Can you work these out from the model? Positions are in its coordinate system, mm. Coordinates: 2 decimals unless noted, no trailing zeros. Write each loop counter-clockwise with the first axis right and the second up, starting at its lowest first coordinate (ties: lowest second). Pieces come first, ordered by that corner, then holes. Notation, with made-up numbers: M 17.25,77.25 L 75.25,77.25 A20 cw 75.25,88.25 Z; hole C 89.25,12.5 d4. An arc over 180 degrees is marked long. Answer as a JSON object with one key per item and string values. Group by question number.
from build123d import *

# Parameters (mm, degrees)
F0_W     = 114.3
F0_H     = 844.55
F0_H_2   = 1968.5
F0_W_2   = 571.5
F0_H_3   = 25.4
F1_DEPTH = 3.175


with BuildPart() as f1:
    # F0 (on Front) → F1 (new body)
    with BuildSketch(Plane.XZ):
        Polygon((-901.7, 0), (0, 0), (0, 2019.3), (-901.7, 2019.3), (-901.7, 1136.65), (-749.3, 1136.65), (-749.3, 882.65), (-901.7, 882.65), align=None)
        with Locations((-819.15, 447.675)):
            Rectangle(F0_W, F0_H, mode=Mode.SUBTRACT)
        Polygon((-736.6, 1354.93125), (-736.6, 1993.9), (-165.1, 1993.9), (-165.1, 1354.93125), (-165.1, 1329.53125), (-165.1, 689.76875), (-165.1, 664.36875), (-165.1, 25.4), (-736.6, 25.4), (-736.6, 664.36875), (-736.6, 689.76875), (-736.6, 1329.53125), align=None, mode=Mode.SUBTRACT)
        with Locations((-819.15, 1571.625)):
            Rectangle(F0_W, F0_H, mode=Mode.SUBTRACT)
        with Locations((-82.55, 1009.65)):
            Rectangle(F0_W, F0_H_2, mode=Mode.SUBTRACT)
        with Locations((-450.85, 1342.23125)):
            Rectangle(F0_W_2, F0_H_3)
        with Locations((-450.85, 677.06875)):
            Rectangle(F0_W_2, F0_H_3)
    extrude(amount=F1_DEPTH)


solid = f1.part
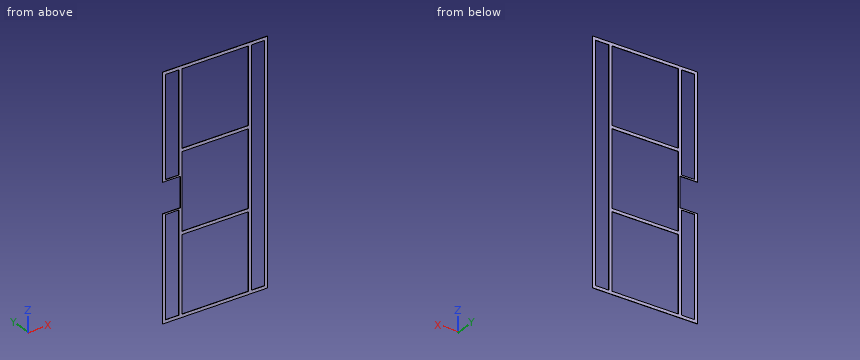
Q1. Please list where these lines run through material, in increasing order: L1, parallel to X at y = -1.6, z = 143; L2, parallel to X at y = -1.1, z = 893; L3, parallel to X at y = -0.6, z = 679.
Q2. If we section it at B-B on z = 594.5: List the corners of the cut face in (x, y) for me (3 decimals), and give its area (3 significant figures).
Q3. Will this pin go through, and if not, where does the flat tip stop? pin 1 (1.6 mm diameter, centred on y = -1.5, z = 1488, fed in from +X).
Q4. If we section it at C-C on y = -1.55: Give the number of separate pieces and of enclosed holes in the cut face, and give its area (3 significant figures).
Q5. If we section it at A-A on x = -247: List the corners of the cut face in (y, z) for me (3 decimals).
Reply:
{
 "1": {"L1": "-901.7 to -876.3, -762 to -736.6, -165.1 to -139.7, -25.4 to 0", "L2": "-749.3 to -736.6, -165.1 to -139.7, -25.4 to 0", "L3": "-901.7 to -876.3, -762 to -139.7, -25.4 to 0"},
 "2": {"outline": "M -901.7,-3.175 L -876.3,-3.175 L -876.3,0 L -901.7,0 Z; M -762,-3.175 L -736.6,-3.175 L -736.6,0 L -762,0 Z; M -165.1,-3.175 L -139.7,-3.175 L -139.7,0 L -165.1,0 Z; M -25.4,-3.175 L 0,-3.175 L 0,0 L -25.4,0 Z", "area": "323 mm^2"},
 "3": {"pin 1": "x = 0"},
 "4": {"separate pieces": "1", "enclosed holes": "6", "area": "268,000 mm^2"},
 "5": {"outline": "M -3.175,0 L 0,0 L 0,25.4 L -3.175,25.4 Z; M -3.175,664.369 L 0,664.369 L 0,689.769 L -3.175,689.769 Z; M -3.175,1329.531 L 0,1329.531 L 0,1354.931 L -3.175,1354.931 Z; M -3.175,1993.9 L 0,1993.9 L 0,2019.3 L -3.175,2019.3 Z"}
}
